The model under review builds one solid part; all positions refer to its coordinate system, in mm. Face numbers are marked on the shaded views. Coordinates: 2 decimals unless noted, no trailing zeros. Order: outer loops, then holes, each group sorted by start corner. A loop starts at its lowest first (then second) coordinate and runs counter-clockwise, first axis right, second up. Notation, with made-up numbers: (3.25, -35) -> (59.25, -35) arc R25 ccw to (59.25, -10) -> close; hole circle Ø11 at (-3.75, -32). An arc over 180 degrees is marked (long way). Put each result on its own line as item: value.
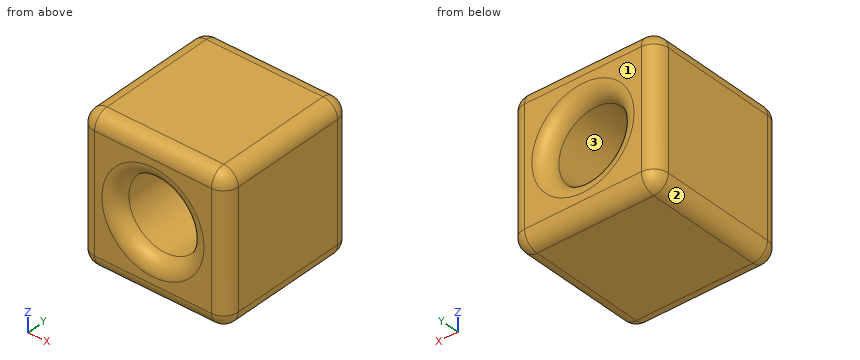
from build123d import *

# Parameters (mm, degrees)
F0_W     = 50
F0_H     = 50
F1_DEPTH = 50
F2_R     = 12.5
F3_DEPTH = 50.001
F4_R     = 5
F5_R     = 5


with BuildPart() as f1:
    # F0 (on Top) → F1 (new body)
    with BuildSketch(Plane.XY):
        Rectangle(F0_W, F0_H)
    extrude(amount=F1_DEPTH)

    # F2 (on face) → F3 (cut, through all)
    with BuildSketch(Plane.XZ.offset(25)):
        with Locations((0, 25)):
            Circle(F2_R)
    extrude(amount=-F3_DEPTH, mode=Mode.SUBTRACT)

    # F4
    f4_edges = [f1.edges().sort_by_distance(p)[0] for p in [
        (0, -25, 50),
        (-25, 0, 50),
        (0, 25, 50),
        (25, 0, 50),
        (25, 25, 25),
        (25, -25, 25),
        (25, 0, 0),
        (0, -25, 0),
        (-25, -25, 25),
        (-25, 0, 0),
        (0, 25, 0),
        (-25, 25, 25),
    ]]
    fillet(f4_edges, radius=F4_R)

    # F5
    f5_edges = [f1.edges().sort_by_distance(p)[0] for p in [
        (-12.5, -25, 25),
        (25, 0, 5),
        (20, 0, 0),
        (0, 20, 0),
        (-12.5, 25, 25),
    ]]
    fillet(f5_edges, radius=F5_R)


solid = f1.part
Item 1: For line 1 (Z direction, x = 0, y = 7); line 2 (Z direction, x = -7.5, y = 3.5); line 3 (X direction, y = -23, z = 31), list the stretches that pass through material, from the lowest coordinate up. Write a range as from..to.
Answers below:
line 1: 0..12.5, 37.5..50
line 2: 0..15, 35..50
line 3: -24..-12.09, 12.09..24
Item 2: Consider section A-A on z = 25. Write out the cut boundary in (x, y), and give its area (3 significant figures).
Answers below:
outline: (-25, -20) arc R5 ccw to (-20, -25) -> (-17.5, -25) arc R5 ccw to (-12.5, -20) -> (-12.5, 20) arc R5 ccw to (-17.5, 25) -> (-20, 25) arc R5 ccw to (-25, 20) -> close; (12.5, -20) arc R5 ccw to (17.5, -25) -> (20, -25) arc R5 ccw to (25, -20) -> (25, 20) arc R5 ccw to (20, 25) -> (17.5, 25) arc R5 ccw to (12.5, 20) -> close
area: 1,210 mm^2
Item 3: Consider section B-B on x = 0. Write out the cut boundary in (y, z), and give its area (3 significant figures).
Answers below:
outline: (-25, 5) arc R5 ccw to (-20, 0) -> (20, 0) arc R5 ccw to (25, 5) -> (25, 7.5) arc R5 ccw to (20, 12.5) -> (-20, 12.5) arc R5 ccw to (-25, 7.5) -> close; (-25, 42.5) arc R5 ccw to (-20, 37.5) -> (20, 37.5) arc R5 ccw to (25, 42.5) -> (25, 45) arc R5 ccw to (20, 50) -> (-20, 50) arc R5 ccw to (-25, 45) -> close
area: 1,210 mm^2
Item 4: Mouldability with a two-part tool opening along X and no side actions: class the marked faces 1, 2 and 3 as +X half, -X half, draft (parallel to the pull), parting line (faces both ways), or undercut.
Answers below:
face 1: draft
face 2: -X half
face 3: undercut
Item 5: Consider section C-C on y = 2. Write out the cut boundary in (x, z).
Answers below:
outline: (-25, 5) arc R5 ccw to (-20, 0) -> (20, 0) arc R5 ccw to (25, 5) -> (25, 45) arc R5 ccw to (20, 50) -> (-20, 50) arc R5 ccw to (-25, 45) -> close; hole circle Ø25 at (0, 25)
Item 6: For pin 1 Ø2 at (x, z) = (-5.5, 12) entering from -Y; pin 2 Ø6 at (x, z) = (-9, 36) entering from -Y, all flat-tipped, find the tip position at first contact; note any pin that passes through.
Answers below:
pin 1: y = -24.39
pin 2: y = -24.99
